Here's how the part is built. I have some questions about the finished solid (model axes, mm). Face numbers are marked on the shaded views. A direction names the side the tool comes from. Coordinates: 2 decimals unless noted, no trailing zeros. Write each loop counter-clockwise with the first axis right and the second up, starting at its lowest first coordinate (ties: lowest second). Pieces come first, ordered by that corner, then holes.
Item 1: I want a section at C-C (y = 21). Please give me the cut outline in (x, z).
Item 2: I want a section at D-D (z = 8.5). Please give me the cut outline in (x, y).
Item 3: If we mould it in two halves opening along Y, with no side actions, what happens to the marked faces 1, 2, 3 and 4? For each: pulls with the +Y half, pulls with the -Y half, needs draft (parallel to the pull), parting line crosses it, or undercut.
Item 4: For the marked faces 5, 6 and 7, which set-ups out of +Z, -Z, +X, -X, +Y, -Y let a thin tool reach every point of the face, with its end or its side?
Item 5: I want a section at A-A (x = 0). Please give me the cut outline in (y, z).
Item 6: I want a section at B-B (z = 26.5). Please give me the cut outline in (x, y), and give its area (3 significant figures).
Item 7: I'm going to push flat-ended pins straight in: P1, Ø9.5, axis at x = 52, y = 13, coming from the +Z side; P2, Ø8, axis at y = 32.5, z = 19.5, coming from the -X side; P3, Ø5, axis at y = 23.5, z = 34, coming from the -X side. Where does each tip first touch, or does it pass through?
Item 8: Please list where these lines run through material, in increasing order: line 1 (X direction, y = 19, z = 9); line 2 (Y direction, x = -44.45, z = 10.25); line 3 (Z direction, x = 0.5, y = 10).
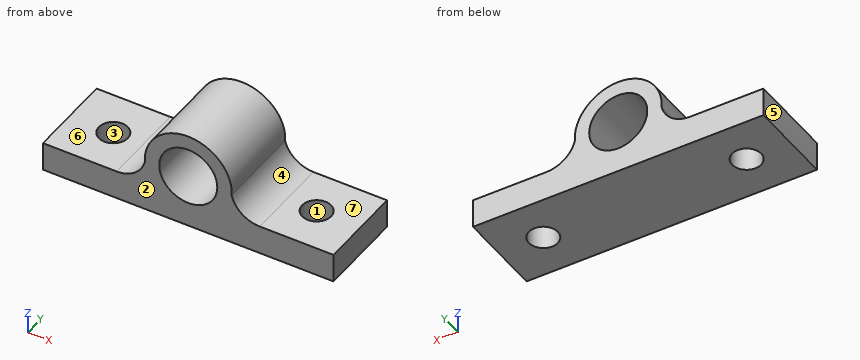
from build123d import *

# Parameters (mm, degrees)
F0_R     = 12.7
F1_DEPTH = 38.1
F2_R     = 6.35
F3_DEPTH = 25.4


with BuildPart() as f1:
    # F0 (on Front) → F1 (new body)
    with BuildSketch(Plane.XZ):
        with BuildLine():
            Line((-63.5, 12.7), (-63.5, 0))
            Line((-63.5, 0), (63.5, 0))
            Line((63.5, 0), (63.5, 12.7))
            Line((63.5, 12.7), (31.315128, 12.7))
            ThreePointArc((31.315128, 12.7), (23.522863, 15.37151), (19.008884, 22.26211))
            ThreePointArc((19.008884, 22.26211), (0, 42.563047), (-19.008884, 22.26211))
            ThreePointArc((-19.008884, 22.26211), (-23.522863, 15.37151), (-31.315128, 12.7))
            Line((-31.315128, 12.7), (-63.5, 12.7))
        make_face()
        with Locations((0, 23.513047)):
            Circle(F0_R, mode=Mode.SUBTRACT)
    extrude(amount=-F1_DEPTH)

    # F2 (on face) → F3 (cut)
    with BuildSketch(Plane.XY.offset(12.7)):
        with Locations((-44.45, 19.05)):
            Circle(F2_R)
        with Locations((44.45, 19.05)):
            Circle(F2_R)
    extrude(amount=-F3_DEPTH, mode=Mode.SUBTRACT)


solid = f1.part
Answer:
1. outline: (-63.5, 0) - (-50.49, 0) - (-50.49, 12.7) - (-63.5, 12.7) - close; (-38.41, 0) - (38.41, 0) - (38.41, 12.7) - (31.32, 12.7) arc R12.7 cw to (19.01, 22.26) arc R19.05 ccw (long way) to (-19.01, 22.26) arc R12.7 cw to (-31.32, 12.7) - (-38.41, 12.7) - close; (50.49, 0) - (63.5, 0) - (63.5, 12.7) - (50.49, 12.7) - close; hole circle Ø25.4 at (0, 23.51)
2. outline: (-63.5, 0) - (63.5, 0) - (63.5, 38.1) - (-63.5, 38.1) - close; hole circle Ø12.7 at (-44.45, 19.05); hole circle Ø12.7 at (44.45, 19.05)
3. face 1: undercut
3. face 2: pulls with the -Y half
3. face 3: undercut
3. face 4: needs draft
4. face 5: +Z, -Z, -X, +Y, -Y
4. face 6: +Z, -X, +Y, -Y
4. face 7: +Z, +X, +Y, -Y
5. outline: (0, 0) - (38.1, 0) - (38.1, 10.81) - (0, 10.81) - close; (0, 36.21) - (38.1, 36.21) - (38.1, 42.56) - (0, 42.56) - close
6. outline: (-18.81, 0) - (-12.34, 0) - (-12.34, 38.1) - (-18.81, 38.1) - close; (12.34, 0) - (18.81, 0) - (18.81, 38.1) - (12.34, 38.1) - close
6. area: 493 mm2
7. P1: stops at z = 12.7
7. P2: stops at x = -23.36
7. P3: stops at x = -17.29
8. line 1: x = -63.5 to -50.8, -38.1 to 38.1, 50.8 to 63.5
8. line 2: y = 0 to 12.7, 25.4 to 38.1
8. line 3: z = 0 to 10.82, 36.2 to 42.56
